Here's how the part is built. I have some questions about the finished solid (model axes, mm). Give positions to 0.01 mm unless a question says otherwise; leave off trailing zeros. Order: outer loops, then holes, each group sorted by start corner. A loop starts at its lowest first (then second) coordinate and runs counter-clockwise, first axis right, second up. Notation, with made-up numbers: M 73.25,-10.75 L 129.25,-10.75 A23 cw 129.25,14.25 Z; hole C 62,56.5 d2. An arc over 180 degrees is marked long. Use one line per item in the form item = value.
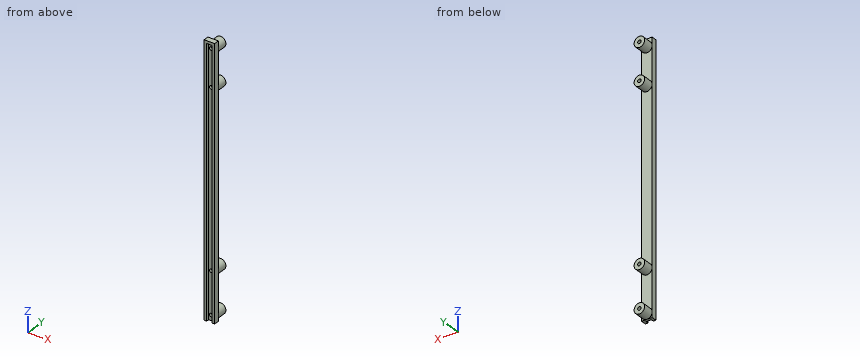
Autodesk Inventor part; units mm, degrees
ref_plane "YZ Plane" through (0, 0, 0) normal (1, 0, 0) x (0, 1, 0)
ref_plane "XZ Plane" through (0, 0, 0) normal (0, 1, 0) x (-1, 0, 0)
ref_plane "XY Plane" through (0, 0, 0) normal (0, 0, 1) x (1, 0, 0)
sketch "Sketch1" plane through (0, 0, 0) normal (0, 1, 0) x (-1, 0, 0)
  line L0 (6.35, 0) -> (-6.35, 0)
  line L1 (-6.35, 0) -> (-6.35, -317.5)
  line L2 (-6.35, -317.5) -> (6.35, -317.5)
  line L3 (6.35, -317.5) -> (6.35, 0)
  circle A0 centre (0, -6.35) radius 2.0955
  circle A1 centre (0, -311.15) radius 2.0955
  circle A2 centre (0, -50.8) radius 2.0955
  circle A3 centre (0, -260.35) radius 2.0955
  point P0 (0, 0)
  dimension "d0" = 12.7
  dimension "d1" = 317.5
  dimension "d2" = 4.191
extrude "Extrusion1" add sketch "Sketch1" against normal blind 6.35
sketch "Sketch2" plane through (0, -6.35, 0) normal (0, -1, 0) x (1, 0, 0)
  line L0 (6.35, 0) -> (-6.35, 0)
  line L1 (-3.175, 0) -> (3.175, 0)
  line L2 (3.175, 0) -> (3.175, -317.5)
  line L3 (3.175, -317.5) -> (-3.175, -317.5)
  line L4 (-3.175, -317.5) -> (-3.175, 0)
  point P0 (0, 0)
extrude "Extrusion2" cut sketch "Sketch2" against normal blind 3.175
sketch "Sketch3" plane through (0, 0, 0) normal (0, 1, 0) x (1, 0, 0)
  circle A0 centre (0, 6.35) radius 6.35
  circle A1 centre (0, 50.8) radius 6.35
  line L0 (-6.35, 317.5) -> (-6.35, 0)
  circle A2 centre (0, 260.35) radius 6.35
  circle A3 centre (0, 311.15) radius 6.35
  circle A4 centre (0, 50.8) radius 2.0955
  circle A5 centre (0, 6.35) radius 2.0955
  circle A6 centre (0, 260.35) radius 2.0955
  circle A7 centre (0, 311.15) radius 2.0955
  point P0 (0, 0)
extrude "Extrusion3" add sketch "Sketch3" along normal blind 12.7
sketch "Sketch4" plane through (6.35, -6.35, 0) normal (0, 0, 1) x (1, 0, 0)
  line L0 (0, 6.35) -> (0, 0)
  line L1 (0, 0) -> (-12.7, 0)
  line L2 (-12.7, 0) -> (-12.7, 6.35)
  line L3 (-12.7, 6.35) -> (0, 6.35)
  line L4 (0, 6.35) -> (0, 0)
  point P0 (-6.35, 6.35)
extrude "Extrusion4" add sketch "Sketch4" along normal blind 3.175
properties part number "HS MOGO Ramp Jig"
Q1. I'm going to push flat-ended pins straight in: pin 1 Ø1 at (x, y) = (0.5, 9.5) entering from +Z; pin 2 Ø1.6 at (x, y) = (-0.5, -4.5) entering from -Z; pin 3 Ø4 at (x, z) = (1, -117) entering from +Y; pin 4 Ø2.5 at (x, z) = (0, -260.35) entering from +Y. Where does each tip first touch, or does it pass through?
Found:
pin_1 = 0
pin_2 = 0
pin_3 = 0
pin_4 = through
Q2. I want a section at B-B on z = -128. Write out the boundary of the cut face in (x, y) (3 decimals).
Found:
outline = M -6.35,-6.35 L -3.175,-6.35 L -3.175,-3.175 L 3.175,-3.175 L 3.175,-6.35 L 6.35,-6.35 L 6.35,0 L -6.35,0 Z
Q3. I need wall thicknesses on L1, parallel to Z at x = 0, y = -2.45 (1 decimal); L2, parallel to X at y = -2.05, z = -6.35. Which ranges of each line are inside material? Lowest first, please.
Found:
L1 = -317.5 to -313.2, -309.1 to -262.4, -258.3 to -52.9, -48.7 to -8.4, -4.3 to 3.2
L2 = -6.35 to -2.1, 2.1 to 6.35
Q4. I want a section at A-A on y = 10. Write out the boundary of the cut face in (x, z), then the cut area to 3 significant figures.
Found:
outline = C 0,-311.15 d12.7; C 0,-260.35 d12.7; C 0,-50.8 d12.7; C 0,-6.35 d12.7; hole C 0,-311.15 d4.19; hole C 0,-260.35 d4.19; hole C 0,-50.8 d4.19; hole C 0,-6.35 d4.19
area = 452 mm²
